Autodesk Inventor part; units mm, degrees
ref_plane "YZ Plane" through (0, 0, 0) normal (1, 0, 0) x (0, 1, 0)
ref_plane "XZ Plane" through (0, 0, 0) normal (0, 1, 0) x (-1, 0, 0)
ref_plane "XY Plane" through (0, 0, 0) normal (0, 0, 1) x (1, 0, 0)
sketch "Sketch1" plane through (0, 0, 0) normal (0, 0, 1) x (1, 0, 0)
  line L0 (90.3787, -90.3787) -> (-349.6213, -90.3787)
  line L1 (-349.6213, -90.3787) -> (-349.6213, -430.3787)
  line L2 (-349.6213, -430.3787) -> (90.3787, -430.3787)
  line L3 (90.3787, -430.3787) -> (90.3787, -90.3787)
  point P0 (0, 0)
  dimension "d0" = 440
  dimension "d1" = 340
extrude "Extrusion1" add sketch "Sketch1" along normal blind 45
sketch "Sketch2" plane through (0, 0, 45) normal (0, 0, 1) x (1, 0, 0)
  line L0 (-334.6213, -105.3787) -> (75.3787, -105.3787)
  line L1 (75.3787, -105.3787) -> (75.3787, -415.3787)
  line L2 (75.3787, -415.3787) -> (-334.6213, -415.3787)
  line L3 (-334.6213, -415.3787) -> (-334.6213, -105.3787)
  line L4 (90.3787, -430.3787) -> (90.3787, -90.3787)
  line L5 (90.3787, -90.3787) -> (-349.6213, -90.3787)
  point P0 (0, 0)
  dimension "d4" = 410
  dimension "d5" = 310
  dimension "d6" = 15
  dimension "d7" = 15
extrude "Extrusion2" cut sketch "Sketch2" against normal blind 5
sketch "Sketch3" plane through (0, 0, 0) normal (0, 0, -1) x (-1, 0, 0)
  line L0 (-35.3787, -145.3787) -> (294.6213, -145.3787)
  line L1 (294.6213, -145.3787) -> (294.6213, -375.3787)
  line L2 (294.6213, -375.3787) -> (-35.3787, -375.3787)
  line L3 (-35.3787, -375.3787) -> (-35.3787, -145.3787)
  line L4 (349.6213, -430.3787) -> (-90.3787, -430.3787)
  line L5 (-90.3787, -430.3787) -> (-90.3787, -90.3787)
  point P0 (0, 0)
  dimension "d10" = 330
  dimension "d11" = 230
  dimension "d12" = 55
  dimension "d13" = 55
extrude "Extrusion3" add sketch "Sketch3" along normal blind 42
properties part number "Monitor"
Here's how the part is built. I have some questions about the finished solid (model axes, mm). A direction names the side the tool comes from. Give positions to 0.01 mm unless a question says otherwise; leave off trailing zeros. Write each loop counter-clockwise with the first axis right and the second up, starting at its lowest first coordinate (ties: lowest second). Pieces come first, ordered by that corner, then holes.
(1) Imagine slicing it at B-B, the plane y = -400. Write out the boundary of the cut face in (x, z).
Output values:
outline: (-349.62, 0) - (90.38, 0) - (90.38, 45) - (75.38, 45) - (75.38, 40) - (-334.62, 40) - (-334.62, 45) - (-349.62, 45) - close
(2) Imagine slicing it at C-C, the plane z = -21.5. Write out the boundary of the cut face in (x, y), and give its area (3 significant figures).
Output values:
outline: (-294.62, -375.38) - (35.38, -375.38) - (35.38, -145.38) - (-294.62, -145.38) - close
area: 75,900 mm2
(3) Will these pins go through, and if not, where does the flat tip stop? pin 1 (12.5 mm diameter, centred on x = -59, z = -22.5, fed in from -Y); pin 2 (3 mm diameter, centred on y = -155.5, z = -7, fed in from -X); pin 3 (10 mm diameter, centred on y = -205, z = -27, fed in from +X).
Output values:
pin 1: stops at y = -375.38
pin 2: stops at x = -294.62
pin 3: stops at x = 35.38
(4) Imagine slicing it at A-A, the plane x = 61. Write out the boundary of the cut face in (y, z).
Output values:
outline: (-430.38, 0) - (-90.38, 0) - (-90.38, 45) - (-105.38, 45) - (-105.38, 40) - (-415.38, 40) - (-415.38, 45) - (-430.38, 45) - close
(5) Thinking about a two-plate mould opening in X: for faces 4 (the face through (-294.621, -259, -21)), 5 (the face through (-132, -258, 40)), 6 (the face through (-132, -375.379, -21)), which applies, pulls with the +X half, pulls with the -X half, needs draft (parallel to the pull), parting line crosses it, or undercut?
Output values:
face 4: pulls with the -X half
face 5: undercut
face 6: needs draft
(6) If I drill on L1, parallel to X at y = -130.5, z = 40.5; L2, parallel to Z at x = 19, y = -224.5; L3, parallel to X at y = -360.5, z = -4, over which ranges is the centre line in solid material (lowest first)?
Output values:
L1: x = -349.62 to -334.62, 75.38 to 90.38
L2: z = -42 to 40
L3: x = -294.62 to 35.38
(7) Imagine slicing it at D-D, the plane x = -28. Write out the boundary of the cut face in (y, z), and give its area (3 significant figures).
Output values:
outline: (-430.38, 0) - (-375.38, 0) - (-375.38, -42) - (-145.38, -42) - (-145.38, 0) - (-90.38, 0) - (-90.38, 45) - (-105.38, 45) - (-105.38, 40) - (-415.38, 40) - (-415.38, 45) - (-430.38, 45) - close
area: 23,400 mm2
(8) On a 3-axis mill with a long thin cutter (end or side, diameter ignored), from which of +Z, -Z, +X, -X, +Y, -Y can I reach the whole of each face in a straight line? I mean faces 1 (the face through (-349.621, -258, 22)), 2 (the face through (-127, -145.379, -21)), 3 (the face through (35.379, -262, -21)). Say none if no direction works.
Output values:
face 1: +Z, -Z, -X, +Y, -Y
face 2: -Z, +X, -X, +Y
face 3: -Z, +X, +Y, -Y
